Geometry check sheet. Reference: the model listing, model coordinates, mm. A direction names the side the tool comes from. Give positions to 0.01 mm unless a question says otherwise; leave off trailing zeros. Write each loop counter-clockwise with the first axis right and the second up, starting at its lowest first coordinate (ties: lowest second). Pieces come first, ordered by that corner, then holes.
(1) Depth check by flat-ended pin: P1, Ø2, axis at y = -5.5, z = 8.5, coming from the -X side; P2, Ø4, axis at x = -4, y = -5.5, coming from the +Z side; P3, Ø3, axis at x = -4.5, z = 1.5, coming from the -Y side. Enter the tip coordinate at first touch or a pass-through.
(2) Tool access check on faces 1 (the cylindrical face through (4.57, 7.167, 7.493)), 2 (the flat face through (-4.5, -7.4, 7)). Record the directions out of +Z, -Z, +X, -X, +Y, -Y that give a thin tool (end or side, any length) a straight path to the whole face; none if there is none.
(3) Thickness scan on line 1 along Y through (x, z) = (0, 7.4); line 2 along Y through (x, z) = (0, 5.25); line 3 along X through (y, z) = (0, 3.25). Record the ranges inside material, lowest first.
(4) Cross-section at A-A (x = 0). Record the boundary of the cut face in (y, z).
```python
from build123d import *

# Parameters (mm, degrees)
CYLINDER009_R     = 2
CYLINDER009_DEPTH = 10
CYLINDER010_R     = 2
CYLINDER010_DEPTH = 10
BOX_W             = 4
BOX_H             = 20
BOX_DEPTH         = 10
CYLINDER004_R     = 8.5
CYLINDER004_DEPTH = 3
CYLINDER005_R     = 10.1
CYLINDER005_DEPTH = 10
CYLINDER002_R     = 15
CYLINDER002_DEPTH = 10
FILLET_R          = 2
FILLET001_R       = 2
FILLET004_R       = 1


with BuildPart() as cylinder009:
    # Cylinder009 → Cylinder009 (new body)
    with BuildSketch(Plane(origin=(0, -12.25, 0), x_dir=(1, 0, 0), z_dir=(0, 0, 1))):
        Circle(CYLINDER009_R)
    extrude(amount=CYLINDER009_DEPTH)


with BuildPart() as fusion003:
    # Cylinder010 → Cylinder010 (new body)
    with BuildSketch(Plane(origin=(0, 12.25, 0), x_dir=(1, 0, 0), z_dir=(0, 0, 1))):
        Circle(CYLINDER010_R)
    extrude(amount=CYLINDER010_DEPTH)

    # Fusion003: union Cylinder009
    add(cylinder009.part)


with BuildPart() as cube:
    # Box → Box (new body)
    with BuildSketch(Plane(origin=(13, -10, 0), x_dir=(1, 0, 0), z_dir=(0, 0, 1))):
        with Locations((2, 10)):
            Rectangle(BOX_W, BOX_H)
    extrude(amount=BOX_DEPTH)


with BuildPart() as cylinder004:
    # Cylinder004 → Cylinder004 (new body)
    with BuildSketch(Plane.XY):
        Circle(CYLINDER004_R)
    extrude(amount=CYLINDER004_DEPTH)


with BuildPart() as fusion001:
    # Cylinder005 → Cylinder005 (new body)
    with BuildSketch(Plane.XY.offset(-10)):
        Circle(CYLINDER005_R)
    extrude(amount=CYLINDER005_DEPTH)

    # Fusion001: union Cylinder004
    add(cylinder004.part)


with BuildPart() as fusion001_1:
    # Fusion001 placement: moved
    add(fusion001.part.moved(Location((0, 0, 7))))


with BuildPart() as obj1:
    # Cylinder002 → Cylinder002 (new body)
    with BuildSketch(Plane.XY):
        Circle(CYLINDER002_R)
    extrude(amount=CYLINDER002_DEPTH)

    # Cut: cut Fusion001
    add(fusion001_1.part, mode=Mode.SUBTRACT)

    # Fillet
    fillet_edges = [obj1.edges().sort_by_distance(p)[0] for p in [
        (-8.5, 0, 10),
    ]]
    fillet(fillet_edges, radius=FILLET_R)

    # Fillet001
    fillet001_edges = [obj1.edges().sort_by_distance(p)[0] for p in [
        (-15, 0, 10),
    ]]
    fillet(fillet001_edges, radius=FILLET001_R)

    # Cut002: cut Cube
    add(cube.part, mode=Mode.SUBTRACT)

    # Fillet004
    fillet004_edges = [obj1.edges().sort_by_distance(p)[0] for p in [
        (13, 4.143485, 9.893358),
        (13, -4.143485, 9.893358),
        (13, 7.483315, 4),
        (13, -7.483315, 4),
    ]]
    fillet(fillet004_edges, radius=FILLET004_R)

    # Cut005: cut Fusion003
    add(fusion003.part, mode=Mode.SUBTRACT)


solid = obj1.part
```
Reply:
1. P1: stops at x = -14.28
1. P2: stops at z = 9.05
1. P3: stops at y = -14.7
2. face 1: +Z, -Z
2. face 2: -Z
3. line 1: y = -15 to -14.25, -10.25 to -8.5, 8.5 to 10.25, 14.25 to 15
3. line 2: y = -15 to -14.25, -10.25 to -10.1, 10.1 to 10.25, 14.25 to 15
3. line 3: x = -15 to -10.1, 10.1 to 13
4. outline: (-15, 0) - (-14.25, 0) - (-14.25, 9.56) arc R2 ccw to (-15, 8) - close; (-10.25, 0) - (-10.1, 0) - (-10.1, 7) - (-8.5, 7) - (-8.5, 8) arc R2 ccw to (-10.25, 9.98) - close; (8.5, 7) - (10.1, 7) - (10.1, 0) - (10.25, 0) - (10.25, 9.98) arc R2 ccw to (8.5, 8) - close; (14.25, 0) - (15, 0) - (15, 8) arc R2 ccw to (14.25, 9.56) - close
